The model under review builds one solid part; all positions refer to its coordinate system, in mm. Face numbers are marked on the shaded views. A direction names the side the tool comes from. Give positions to 0.01 mm unless a question says otherwise; leave off trailing zeros. Write each loop counter-clockwise with the first axis right and the second up, starting at its lowest first coordinate (ties: lowest second). Pieces come first, ordered by that corner, then holes. Notation, with made-up numbers: (55, -1) - (109, -1) arc R20 cw to (109, 35) - close; hole circle Ø2 at (85.25, -9). An arc over 180 degrees is marked (long way). Write item = value, one per line.
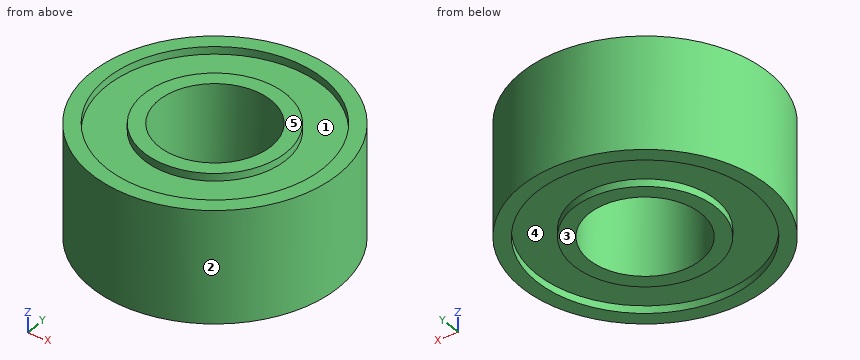
```python
from build123d import *

# Parameters (mm, degrees)
SKETCH1_R           = 9.5
SKETCH1_R_2         = 7.5
BOSS_EXTRUDE1_DEPTH = 7.5
SKETCH4_R           = 14.5
SKETCH4_R_2         = 9.5
BOSS_EXTRUDE2_DEPTH = 6.5
SKETCH5_R           = 16.5
SKETCH5_R_2         = 14.5
BOSS_EXTRUDE3_DEPTH = 7.5


with BuildPart() as part:
    # Sketch1 → Boss-Extrude1 (new, symmetric)
    with BuildSketch(Plane.XY):
        Circle(SKETCH1_R)
        Circle(SKETCH1_R_2, mode=Mode.SUBTRACT)
    extrude(amount=BOSS_EXTRUDE1_DEPTH, both=True)

    # Sketch4 → Boss-Extrude2 (add, symmetric)
    with BuildSketch(Plane.XY):
        with Locations(Location((0, 0, 0), (0, 0, 180))):
            Circle(SKETCH4_R)
        Circle(SKETCH4_R_2, mode=Mode.SUBTRACT)
    extrude(amount=BOSS_EXTRUDE2_DEPTH, both=True)

    # Sketch5 → Boss-Extrude3 (add, symmetric)
    with BuildSketch(Plane.XY):
        Circle(SKETCH5_R)
        Circle(SKETCH5_R_2, mode=Mode.SUBTRACT)
    extrude(amount=BOSS_EXTRUDE3_DEPTH, both=True)


solid = part.part
```
1. For line 1 (Y direction, x = 0, z = -1.75); line 2 (Y direction, x = 0, z = -7.25); line 3 (X direction, y = 1.5, z = -7), list the stretches that pass through material, from the lowest coordinate up. Write a range as from..to.
Findings below:
line_1 = -16.5..-7.5, 7.5..16.5
line_2 = -16.5..-14.5, -9.5..-7.5, 7.5..9.5, 14.5..16.5
line_3 = -16.43..-14.42, -9.38..-7.35, 7.35..9.38, 14.42..16.43
2. Draft analysis for pull direction X (two halves, no side actions). For the marked faces 1, 2 and 3, state which applies: +X half, -X half, draft (parallel to the pull), parting line (faces both ways), or undercut.
Findings below:
face_1 = undercut
face_2 = parting line
face_3 = draft
3. Insertion check: P1, Ø2, axis at x = -9, y = 8, coming from the -Z side; P2, Ø8, axis at x = 11, z = -5.5, coming from the +Y side; P3, Ø1.5, axis at x = -9.5, z = -4.5, coming from the -Y side. Each pin has a flat end and moves straight along its axis. Give the tip position at first contact, or say it passes through.
Findings below:
P1 = -6.5
P2 = 14.94
P3 = -13.99
4. Machinability: for the marked faces 4 and 5, which of the approach directions +Z, -Z, +X, -X, +Y, -Y give a long, thin tool a straight path to every point of the face, cutting with its end or side? Answer none if there is none.
Findings below:
face_4 = -Z
face_5 = +Z, +X, -X, +Y, -Y
5. Take a section at C-C on z = 1.5. Give the boundary of the cut face in (x, y).
Findings below:
outline = circle Ø33 at (0, 0); hole circle Ø15 at (0, 0)
6. Take a section at D-D on y = 11. Give the boundary of the cut face in (x, z), and give its area (3 significant figures).
Findings below:
outline = (-12.3, -7.5) - (-9.45, -7.5) - (-9.45, -6.5) - (9.45, -6.5) - (9.45, -7.5) - (12.3, -7.5) - (12.3, 7.5) - (9.45, 7.5) - (9.45, 6.5) - (-9.45, 6.5) - (-9.45, 7.5) - (-12.3, 7.5) - close
area = 331 mm²
7. Take a section at A-A on y = 0. Give the boundary of the cut face in (x, z), and give its area (3 significant figures).
Findings below:
outline = (-16.5, -7.5) - (-14.5, -7.5) - (-14.5, -6.5) - (-9.5, -6.5) - (-9.5, -7.5) - (-7.5, -7.5) - (-7.5, 7.5) - (-9.5, 7.5) - (-9.5, 6.5) - (-14.5, 6.5) - (-14.5, 7.5) - (-16.5, 7.5) - close; (7.5, -7.5) - (9.5, -7.5) - (9.5, -6.5) - (14.5, -6.5) - (14.5, -7.5) - (16.5, -7.5) - (16.5, 7.5) - (14.5, 7.5) - (14.5, 6.5) - (9.5, 6.5) - (9.5, 7.5) - (7.5, 7.5) - close
area = 250 mm²
